Here's how the part is built. I have some questions about the finished solid (model axes, mm). A direction names the side the tool comes from. Coordinates: 2 decimals unless noted, no trailing zeros. Loops run counter-clockwise (first coordinate to the right, second up) from the corner with the lowest first, then second, coordinate; pieces in that order, holes last.
from build123d import *

# Parameters (mm, degrees)
SKETCH1_W                 = 80
SKETCH1_H                 = 14.75
BOSS_EXTRUDE1_DEPTH       = 28.5
SKETCH7_W                 = 25.5
SKETCH7_H                 = 10
CUT_EXTRUDE3_DEPTH        = 86.244592937
M4X0_7_TAPPED_HOLE3_D     = 3.3
M4X0_7_TAPPED_HOLE3_DEPTH = 1.5
M4_CLEARANCE_HOLE1_D      = 4.5
M4_CLEARANCE_HOLE1_DEPTH  = 1.5
SKETCH15_R                = 40
CUT_EXTRUDE4_DEPTH        = 50.665285915
BOSS_EXTRUDE3_START       = -4.75
SKETCH19_W                = 10.25
SKETCH19_H                = 13
SKETCH19_H_2              = 14.5
BOSS_EXTRUDE3_DEPTH       = 4.75
M4_CLEARANCE_HOLE3_D      = 4.5


with BuildPart() as part:
    # Sketch1 → Boss-Extrude1 (new body)
    with BuildSketch(Plane.XY):
        Rectangle(SKETCH1_W, SKETCH1_H)
    extrude(amount=BOSS_EXTRUDE1_DEPTH)

    # Sketch7 → Cut-Extrude3 (cut, through all)
    with BuildSketch(Plane.ZY.offset(40)):
        with Locations((14.25, 2.375)):
            Rectangle(SKETCH7_W, SKETCH7_H)
    extrude(amount=-CUT_EXTRUDE3_DEPTH, mode=Mode.SUBTRACT)

    # M4x0.7 Tapped Hole3
    with Locations(Plane.XY.offset(1.5)):
        with Locations((-35.75, 1.875), (35.75, 1.875)):
            Hole(M4X0_7_TAPPED_HOLE3_D / 2, depth=M4X0_7_TAPPED_HOLE3_DEPTH)

    # M4 Clearance Hole1
    with Locations(Plane(origin=(0, 0, 27), x_dir=(-1, 0, 0), z_dir=(0, 0, -1))):
        with Locations((-35.75, 1.875), (35.75, 1.875)):
            Hole(M4_CLEARANCE_HOLE1_D / 2, depth=M4_CLEARANCE_HOLE1_DEPTH)

    # Sketch15 → Cut-Extrude4 (cut, through all)
    with BuildSketch(Plane.XY.offset(28.5)):
        with Locations((0, 37.625)):
            Circle(SKETCH15_R)
    extrude(amount=-CUT_EXTRUDE4_DEPTH, mode=Mode.SUBTRACT)

    # Sketch19 → Boss-Extrude3 (add)
    with BuildSketch(Plane.XZ.offset(7.375).offset(BOSS_EXTRUDE3_START)):
        with Locations((-45.125, 22)):
            Rectangle(SKETCH19_W, SKETCH19_H)
        with Locations((45.125, 7.25)):
            Rectangle(SKETCH19_W, SKETCH19_H_2)
    extrude(amount=BOSS_EXTRUDE3_DEPTH)

    # M4 Clearance Hole3 (through all)
    with Locations(Plane(origin=(0, -2.625, 0), x_dir=(1, 0, 0), z_dir=(0, 1, 0))):
        with Locations((-45.25, -25), (45.25, -5)):
            Hole(M4_CLEARANCE_HOLE3_D / 2)


solid = part.part
Q1. Suppose I cut it at C-C on y = -5.5. Write out the boundary of the cut face in (x, z).
Q2. Will these pins go through, and if not, where does the flat tip stop? P1, Ø1.6, axis at y = 0, z = 27.5, coming from the -X side; P2, Ø4, axis at x = 45.25, z = 5, coming from the -Y side; P3, Ø2.5, axis at x = -44, y = -6, coming from the -Z side; P4, Ø4, axis at x = 43, y = -5, coming from the +Z side.
Q3. Please list where these lines run through material, in increasing order: probe 1 along Y at (x, z) = (-35.75, 0.3) (3 decimals); probe 2 along Z at (x, y) = (28, 5); probe 3 along Y at (x, z) = (-35.75, 28.15) (3 decimals).
Q4. Suppose I cut it at A-A on z = 5. Write out the boundary of the cut face in (x, y) (3 decimals), and give its area (3 significant figures).
Q5. Suppose I cut it at B-B on x = -45.25. Write out the boundary of the cut face in (y, z) (3 decimals), and give its area (3 significant figures).
Q6. We'd pull the mould along Z, two halves only. Please class faces 4 (the cylindrical face through (-43.464, -5.033, 26.369)), 5 (the cylindrical face through (-33.672, 1.013, 27.76)), 6 (the flat face through (45, -5, 14.5)): pulls with the +Z half, pulls with the -Z half, needs draft (parallel to the pull), parting line crosses it, or undercut.
Q7. Suppose I cut it at D-D on x = 35.75. Write out the boundary of the cut face in (y, z) (3 decimals).
Q8. For faces 1 (the flat face through (8, -2, 27)), 2 (the cylindrical face through (37.828, 1.013, 27.76)), 3 (the flat face through (-40, -3, 6)), which set-ups out of +Z, -Z, +X, -X, +Y, -Y let a thin tool reach every point of the face, with its end or its side?
Check values:
1. outline: (-50.25, 15.5) - (-40, 15.5) - (-40, 0) - (50.25, 0) - (50.25, 14.5) - (40, 14.5) - (40, 28.5) - (-50.25, 28.5) - close; hole circle Ø4.5 at (-45.25, 25); hole circle Ø4.5 at (45.25, 5)
2. P1: stops at x = -40
2. P2: passes through
2. P3: stops at z = 15.5
2. P4: stops at z = 14.5
3. probe 1: y = -7.375 to 0.225, 3.525 to 7.375
3. probe 2: z = 0 to 1.5, 27 to 28.5
3. probe 3: y = -7.375 to -0.375, 4.125 to 7.375
4. outline: (-40, -7.375) - (43, -7.375) - (43, -2.625) - (-40, -2.625) - close; (47.5, -7.375) - (50.25, -7.375) - (50.25, -2.625) - (47.5, -2.625) - close
4. area: 407 mm2
5. outline: (-7.375, 15.5) - (-2.625, 15.5) - (-2.625, 22.75) - (-7.375, 22.75) - close; (-7.375, 27.25) - (-2.625, 27.25) - (-2.625, 28.5) - (-7.375, 28.5) - close
5. area: 40.4 mm2
6. face 4: undercut
6. face 5: needs draft
6. face 6: pulls with the +Z half
7. outline: (-7.375, 0) - (0.225, 0) - (0.225, 1.5) - (-2.625, 1.5) - (-2.625, 27) - (-0.375, 27) - (-0.375, 28.5) - (-7.375, 28.5) - close; (3.525, 0) - (7.375, 0) - (7.375, 1.5) - (3.525, 1.5) - close; (4.125, 27) - (7.375, 27) - (7.375, 28.5) - (4.125, 28.5) - close
8. face 1: +X, -X, +Y
8. face 2: +Z
8. face 3: -Z, -X, +Y, -Y
